```python
from build123d import *

# Parameters (mm, degrees)
SKETCH1_W           = 50
SKETCH1_H           = 70
BOSS_EXTRUDE1_DEPTH = 200
SKETCH2_R           = 5
CUT_EXTRUDE1_DEPTH  = 200
FILLET1_R           = 10


with BuildPart() as part:
    # Sketch1 → Boss-Extrude1 (new body)
    with BuildSketch(Plane(origin=(0, 0, 0), x_dir=(1, 0, 0), z_dir=(0, 1, 0))):
        Rectangle(SKETCH1_W, SKETCH1_H)
    extrude(amount=BOSS_EXTRUDE1_DEPTH)

    # Sketch2 → Cut-Extrude1 (cut)
    with BuildSketch(Plane.ZY.offset(25)):
        with Locations((0, 30)):
            Circle(SKETCH2_R)
    extrude(amount=-CUT_EXTRUDE1_DEPTH, mode=Mode.SUBTRACT)

    # Fillet1
    fillet1_edges = [part.edges().sort_by_distance(p)[0] for p in [
        (0, 0, 35),
        (0, 0, -35),
    ]]
    fillet(fillet1_edges, radius=FILLET1_R)


solid = part.part
```
Source: CAD feature listing. Evaluate the final solid. Frame: model axes, mm. Round coordinates to 2 decimals unless told otherwise and drop trailing zeros. Write each loop counter-clockwise with the first axis right and the second up, starting at its lowest first coordinate (ties: lowest second). Pieces come first, ordered by that corner, then holes. Notation, with made-up numbers: M 17.25,54 L 42.25,54 A17 ccw 42.25,86 Z; hole C 45.25,-10.75 d1. An arc over 180 degrees is marked long. Answer as a JSON object with one key per item and string values. Group by question number.
(1) Section query B-B on y = 30. Output: boundary loops of the cut face in (x, z).
(2) Section query A-A on z = 0. Output: boundary loops of the cut face in (x, y).
(3) First-contact query: pin 1 (6 mm diameter, centred on y = 30, z = 0, fed in from +X). Flat tip, straight axial feed; report the tip coordinate or a pass-through.
(4) Mould query, pull axis Z, two halves, no side actions, for faces 1 (the flat face through (-25, 99, 0)), 2 (the cylindrical face through (0.35, 3.01, 32.15)), 3 (the flat face through (0, 104, -35)), 4 (the cylindrical face through (-0.35, 25.12, -1.08)). Classes: +Z half, -Z half, draft (parallel to the pull), parting line (faces both ways), or undercut.
(5) Ray query, line 1 (Y direction, x = 9, z = 0); line 2 (Y direction, x = 22, z = 1.5); line 3 (Z direction, x = 2.5, y = 34). Return the intervals inside material, ascending. Write a range as [from, to].
Computed values:
{
 "1": {"outline": "M -25,-35 L 25,-35 L 25,-5 L -25,-5 Z; M -25,5 L 25,5 L 25,35 L -25,35 Z"},
 "2": {"outline": "M -25,0 L 25,0 L 25,25 L -25,25 Z; M -25,35 L 25,35 L 25,200 L -25,200 Z"},
 "3": {"pin 1": "through"},
 "4": {"face 1": "draft", "face 2": "+Z half", "face 3": "-Z half", "face 4": "undercut"},
 "5": {"line 1": "[0, 25], [35, 200]", "line 2": "[0, 25.23], [34.77, 200]", "line 3": "[-35, -3], [3, 35]"}
}
